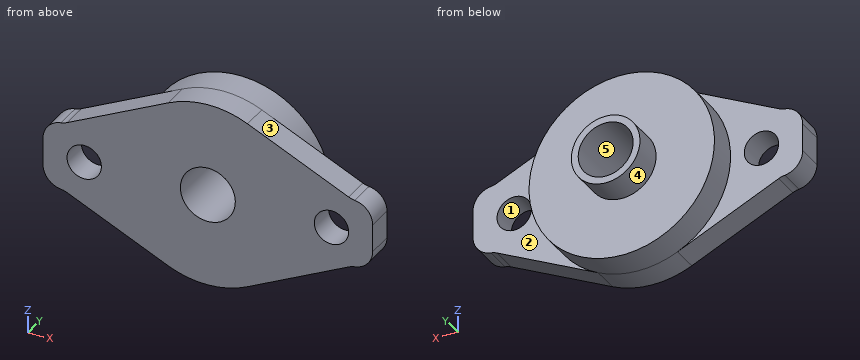
```python
from build123d import *

# Parameters (mm, degrees)
SKETCH_1_R      = 2.5
SKETCH_1_R_2    = 4
EXTRUDE_1_DEPTH = 4
SKETCH_2_R      = 13.5
SKETCH_2_R_2    = 4
EXTRUDE_2_DEPTH = 4.5
SKETCH_3_R      = 5
SKETCH_3_R_2    = 4
EXTRUDE_3_DEPTH = 4.5


with BuildPart() as part:
    # 草图1 → 凸台-拉伸1 (new body)
    with BuildSketch(Plane(origin=(0, 0, 0), x_dir=(1, 0, 0), z_dir=(0, 1, 0))):
        with BuildLine():
            Line((-5.773005503, 12.203376888), (-20.499093296, 5.236962046))
            ThreePointArc((-20.499093296, 5.236962046), (-20.934809728, 5.070925602), (-21.390991704, 4.974411789))
            ThreePointArc((-21.390991704, 4.974411789), (-23.255324268, 3.978259954), (-24, 2))
            Line((-24, 2), (-24, -2))
            ThreePointArc((-24, -2), (-23.255324268, -3.978259954), (-21.390991704, -4.974411789))
            ThreePointArc((-21.390991704, -4.974411789), (-20.934809728, -5.070925602), (-20.499093296, -5.236962046))
            Line((-20.499093296, -5.236962046), (-5.773005503, -12.203376888))
            ThreePointArc((-5.773005503, -12.203376888), (0, -13.5), (5.773005503, -12.203376888))
            Line((5.773005503, -12.203376888), (20.499093296, -5.236962046))
            ThreePointArc((20.499093296, -5.236962046), (20.934809728, -5.070925602), (21.390991704, -4.974411789))
            ThreePointArc((21.390991704, -4.974411789), (23.255324268, -3.978259954), (24, -2))
            Line((24, -2), (24, 2))
            ThreePointArc((24, 2), (23.255324268, 3.978259954), (21.390991704, 4.974411789))
            ThreePointArc((21.390991704, 4.974411789), (20.934809728, 5.070925602), (20.499093296, 5.236962046))
            Line((20.499093296, 5.236962046), (5.773005503, 12.203376888))
            ThreePointArc((5.773005503, 12.203376888), (0, 13.5), (-5.773005503, 12.203376888))
        make_face()
        with Locations(Location((-18, 0, 0), (0, 0, 270))):
            Circle(SKETCH_1_R, mode=Mode.SUBTRACT)
        with Locations(Location((0, 0, 0), (0, 0, 270))):
            Circle(SKETCH_1_R_2, mode=Mode.SUBTRACT)
        with Locations(Location((18, 0, 0), (0, 0, 270))):
            Circle(SKETCH_1_R, mode=Mode.SUBTRACT)
    extrude(amount=EXTRUDE_1_DEPTH)

    # 草图2 → 凸台-拉伸2 (add)
    with BuildSketch(Plane(origin=(0, 4, 0), x_dir=(1, 0, 0), z_dir=(0, 1, 0))):
        with Locations(Location((0, 0, 0), (0, 0, 64.68274989))):
            Circle(SKETCH_2_R)
        with Locations(Location((0, 0, 0), (0, 0, 270))):
            Circle(SKETCH_2_R_2, mode=Mode.SUBTRACT)
    extrude(amount=EXTRUDE_2_DEPTH)

    # 草图3 → 凸台-拉伸3 (add)
    with BuildSketch(Plane(origin=(0, 8.5, 0), x_dir=(1, 0, 0), z_dir=(0, 1, 0))):
        with Locations(Location((0, 0, 0), (0, 0, 270))):
            Circle(SKETCH_3_R)
        with Locations(Location((0, 0, 0), (0, 0, 270))):
            Circle(SKETCH_3_R_2, mode=Mode.SUBTRACT)
    extrude(amount=EXTRUDE_3_DEPTH)


solid = part.part
```
Part model, mm, in its own coordinate system. Face numbers are marked on the shaded views. A direction names the side the tool comes from. Round coordinates to 2 decimals unless told otherwise and drop trailing zeros. Write each loop counter-clockwise with the first axis right and the second up, starting at its lowest first coordinate (ties: lowest second). Pieces come first, ordered by that corner, then holes. Notation, with made-up numbers: M 71,-4.75 L 108,-4.75 A20 cw 108,9.25 Z; hole C 24.5,-29.5 d7. An arc over 180 degrees is marked long. One line per question, with ' | ' between items.
(1) Pin check, flat tips, straight feed: pin 1 (4 mm diameter, centred on x = -18, z = 0, fed in from -Y); pin 2 (5 mm diameter, centred on x = 6, y = 11.5, fed in from -Z); pin 3 (3 mm diameter, centred on x = 7, y = 9, fed in from -Z); pin 4 (9 mm diameter, centred on x = 16.5, z = 0, fed in from +Y). Stop position of each tip, or through.
Answer key:
pin 1: passes through | pin 2: stops at z = -3.57 | pin 3: stops at z = -12.29 | pin 4: stops at y = 8.5
(2) Saw through at D-D on y = 6. Write the cut outline in (x, z), then the cut area to 3 significant figures.
Answer key:
outline: C 0,0 d27; hole C 0,0 d8 | area: 522 mm^2
(3) Probe line 1 along X through (y, z) = (1.1, 0); line 2 along X through (y, z) = (1.75, -1.75); line 3 along Y through (x, z) = (-10, -8.25). List the from-to ranges inside material, lowest first.
Answer key:
line 1: x = -24 to -20.5, -15.5 to -4, 4 to 15.5, 20.5 to 24 | line 2: x = -24 to -19.79, -16.21 to -3.6, 3.6 to 16.21, 19.79 to 24 | line 3: y = 0 to 8.5
(4) 3-axis set-ups, long thin cutter, end or side, ignore diameter. For the marked faces 4 and 5: which of +Z, -Z, +X, -X, +Y, -Y reach the whole face in a straight line?
Answer key:
face 4: +Y | face 5: +Y, -Y
(5) Saw through at B-B on z = 0. Write the cut outline in (x, y), then the cut area to 4 significant figures.
Answer key:
outline: M -24,0 L -20.5,0 L -20.5,4 L -24,4 Z; M -15.5,0 L -4,0 L -4,13 L -5,13 L -5,8.5 L -13.5,8.5 L -13.5,4 L -15.5,4 Z; M 4,0 L 15.5,0 L 15.5,4 L 13.5,4 L 13.5,8.5 L 5,8.5 L 5,13 L 4,13 Z; M 20.5,0 L 24,0 L 24,4 L 20.5,4 Z | area: 214.5 mm^2
(6) Two-plate mould, pull along X, no slides. Class the marked faces 1, 2 and 3: released by +X, released by -X, zero draft, split by the parting line, or undercut.
Answer key:
face 1: undercut | face 2: zero draft | face 3: released by +X
(7) Saw through at A-A on x = 0. Write the cut outline in (y, z).
Answer key:
outline: M 0,-13.5 L 8.5,-13.5 L 8.5,-5 L 13,-5 L 13,-4 L 0,-4 Z; M 0,4 L 13,4 L 13,5 L 8.5,5 L 8.5,13.5 L 0,13.5 Z
(8) Saw through at C-C on y = 1.5. Write the cut outline in (x, z), then the cut area to 3 significant figures.
Answer key:
outline: M -24,-2 A3 ccw -21.39,-4.97 A3 cw -20.5,-5.24 L -5.77,-12.2 A13.5 ccw 5.77,-12.2 L 20.5,-5.24 A3 cw 21.39,-4.97 A3 ccw 24,-2 L 24,2 A3 ccw 21.39,4.97 A3 cw 20.5,5.24 L 5.77,12.2 A13.5 ccw -5.77,12.2 L -20.5,5.24 A3 cw -21.39,4.97 A3 ccw -24,2 Z; hole C -18,0 d5; hole C 0,0 d8; hole C 18,0 d5 | area: 789 mm^2
